CAD build for the part. Positions are in the model's coordinates, mm. A direction names the side the tool comes from. Give positions to 0.01 mm unless a question says otherwise; leave off trailing zeros. Write each loop counter-clockwise with the first axis right and the second up, starting at its lowest first coordinate (ties: lowest second). Pieces come first, ordered by that corner, then holes. Notation, with made-up numbers: (-27, -20.75) -> (-4, -20.75) arc R25 cw to (-4, -2.75) -> close; hole circle Ø5 at (22.5, 15.5). An arc over 180 degrees is marked (long way). Use one line per item in the form item = value. Start each with the question number.
from build123d import *

# Parameters (mm, degrees)
SKETCH1_W          = 2.5
SKETCH1_H          = 49.03
SKETCH1_W_2        = 30
SKETCH1_H_2        = 2.5
CUT_EXTRUDE1_DEPTH = 10


with BuildPart() as part:
    # Sketch1 → Revolve1 (revolve)
    with BuildSketch(Plane.XY, mode=Mode.PRIVATE) as revolve1_sk:
        with Locations((8.376364172, 0.726593752)):
            Rectangle(SKETCH1_W, SKETCH1_H)
        with Locations((-7.873635828, 22.461593752)):
            Rectangle(SKETCH1_W_2, SKETCH1_H_2)
    revolve(revolve1_sk.sketch.rotate(Axis((7.126364172, -23.788406248, 0), (1, 0, 0)), 90), axis=Axis((7.126364172, -23.788406248, 0), (1, 0, 0)))

    # Sketch2 → Cut-Extrude1 (cut)
    with BuildSketch(Plane(origin=(9.626364172, 0, 0), x_dir=(0, 0, -1), z_dir=(1, 0, 0))):
        with BuildLine():
            Line((0, -23.788406248), (0, -18.788406248))
            ThreePointArc((0, -18.788406248), (-5, -23.788406248), (0, -28.788406248))
            Line((0, -28.788406248), (0, -23.788406248))
        make_face()
        with BuildLine():
            ThreePointArc((5, -23.788406248), (3.535533906, -20.252872342), (0, -18.788406248))
            Line((0, -18.788406248), (0, -23.788406248))
            Line((0, -23.788406248), (5, -23.788406248))
        make_face()
        with BuildLine():
            Line((5, -23.788406248), (0, -23.788406248))
            Line((0, -23.788406248), (0, -28.788406248))
            ThreePointArc((0, -28.788406248), (3.535533906, -27.323940154), (5, -23.788406248))
        make_face()
        with BuildLine():
            ThreePointArc((1.25, -53.788406248), (0.883883476, -52.904522772), (0, -52.538406248))
            Line((0, -52.538406248), (0, -55.038406248))
            ThreePointArc((0, -55.038406248), (0.883883476, -54.672289725), (1.25, -53.788406248))
        make_face()
        with BuildLine():
            Line((0, -55.038406248), (0, -52.538406248))
            ThreePointArc((0, -52.538406248), (-1.25, -53.788406248), (0, -55.038406248))
        make_face()
        with BuildLine():
            ThreePointArc((1.25, 6.211593752), (0.883883476, 7.095477228), (0, 7.461593752))
            Line((0, 7.461593752), (0, 4.961593752))
            ThreePointArc((0, 4.961593752), (0.883883476, 5.327710275), (1.25, 6.211593752))
        make_face()
        with BuildLine():
            Line((0, 4.961593752), (0, 7.461593752))
            ThreePointArc((0, 7.461593752), (-1.25, 6.211593752), (0, 4.961593752))
        make_face()
    extrude(amount=-CUT_EXTRUDE1_DEPTH, mode=Mode.SUBTRACT)


solid = part.part
1) Cut at A-A (x = -2). Give the cut face in (y, z).
2) 3-axis set-ups, long thin cutter, end or side, ignore diameter. For faces 4 (the face through (9.626, -24, -10)), 5 (the face through (7.126, -64, 26)): which of +Z, -Z, +X, -X, +Y, -Y reach the whole face in a straight line?
3) Two-plate mould, pull along Z, no slides. Class faces 1 (the face through (-22.874, -6, -42)), 2 (the face through (7.126, -24, -9)), 3 (the face through (-7.664, -38.056, 45.307)): released by +Z, released by -Z, zero draft, split by the parting line, or undercut.
4) Cut at C-C (y = -57.5). Give the cut face in (x, z), and give its area (3 significant figures).
5) Pin check, flat tips, straight feed: pin 1 (12 mm diameter, centred on x = -7, z = -26, fed in from +Y); pin 2 (12 mm diameter, centred on x = 0.5, y = 9.5, fed in from +Z); pin 3 (10 mm diameter, centred on x = 5, z = 15, fed in from +Y). Stop position of each tip, or through.
6) Wall check: line 1 along Y through (x, z) = (-7.5, 0); line 2 along X through (y, z) = (-8.5, -27.5); line 3 along Z through (x, y) = (-17.5, -34). Give the ranges that are in metal, low to high. Write a range as from..to.
7) Cut at B-B (z = 38.5). Give the cut face in (x, y).
Final values:
q1.outline = circle Ø95 at (-23.79, 0); hole circle Ø90 at (-23.79, 0)
q2.face_4 = +Z, -Z, +X, +Y, -Y
q2.face_5 = -X
q3.face_1 = zero draft
q3.face_2 = undercut
q3.face_3 = split by the parting line
q4.outline = (-22.87, -33.46) -> (7.13, -33.46) -> (7.13, -35.6) -> (9.63, -35.6) -> (9.63, 35.6) -> (7.13, 35.6) -> (7.13, 33.46) -> (-22.87, 33.46) -> (-22.87, 29.81) -> (7.13, 29.81) -> (7.13, -29.81) -> (-22.87, -29.81) -> close
q4.area = 397 mm^2
q5.pin_1 = 19.3
q5.pin_2 = 38.88
q5.pin_3 = 24.11
q6.line_1 = -71.29..-68.79, 21.21..23.71
q6.line_2 = 7.13..9.63
q6.line_3 = -46.39..-43.83, 43.83..46.39
q7.outline = (-22.87, -51.61) -> (7.13, -51.61) -> (7.13, -54.15) -> (9.63, -54.15) -> (9.63, 6.57) -> (7.13, 6.57) -> (7.13, 4.03) -> (-22.87, 4.03) -> (-22.87, -0.49) -> (7.13, -0.49) -> (7.13, -47.09) -> (-22.87, -47.09) -> close
